```python
from build123d import *

# Parameters (mm, degrees)
BOSS_EXTRUDE1_DEPTH         = 561.975
F_1_4_20_TAPPED_HOLE1_D     = 5.1054
F_1_4_20_TAPPED_HOLE1_DEPTH = 16.51
F_1_4_20_TAPPED_HOLE1_TIP   = 1.533816902
F_1_4_20_TAPPED_HOLE2_D     = 5.1054
F_1_4_20_TAPPED_HOLE2_DEPTH = 16.51
F_1_4_20_TAPPED_HOLE2_TIP   = 1.533816902


with BuildPart() as part:
    # Sketch1 → Boss-Extrude1 (new body)
    with BuildSketch(Plane.XY):
        Polygon((7.332348419, 0), (3.666174209, 6.35), (-3.666174209, 6.35), (-7.332348419, 0), (-3.666174209, -6.35), (3.666174209, -6.35), align=None)
    extrude(amount=BOSS_EXTRUDE1_DEPTH)

    # 1/4-20 Tapped Hole1
    with Locations(Plane.XY.offset(561.975)):
        with Locations((0, 0)):
            Hole(F_1_4_20_TAPPED_HOLE1_D / 2, depth=F_1_4_20_TAPPED_HOLE1_DEPTH)
            with Locations((0, 0, -(F_1_4_20_TAPPED_HOLE1_DEPTH + F_1_4_20_TAPPED_HOLE1_TIP / 2))):  # 118° drill point
                Cone(0, F_1_4_20_TAPPED_HOLE1_D / 2, F_1_4_20_TAPPED_HOLE1_TIP, mode=Mode.SUBTRACT)

    # 1/4-20 Tapped Hole2
    with Locations(Plane(origin=(0, 0, 0), x_dir=(-1, 0, 0), z_dir=(0, 0, -1))):
        with Locations((0, 0)):
            Hole(F_1_4_20_TAPPED_HOLE2_D / 2, depth=F_1_4_20_TAPPED_HOLE2_DEPTH)
            with Locations((0, 0, -(F_1_4_20_TAPPED_HOLE2_DEPTH + F_1_4_20_TAPPED_HOLE2_TIP / 2))):  # 118° drill point
                Cone(0, F_1_4_20_TAPPED_HOLE2_D / 2, F_1_4_20_TAPPED_HOLE2_TIP, mode=Mode.SUBTRACT)


solid = part.part
```
Source: CAD feature listing. Evaluate the final solid. Frame: model axes, mm. Round coordinates to 2 decimals unless told otherwise and drop trailing zeros. Loops run counter-clockwise (first coordinate to the right, second up) from the corner with the lowest first, then second, coordinate; pieces in that order, holes last. Notation, with made-up numbers: M 15,-15 L 45,-15 A15 ccw 45,0 Z; hole C 42,-40 d2. An arc over 180 degrees is marked long. Use a Markdown table: item, result. Add a question column.
1. Contact query for a flat-ended pin moving along its axis: pin 1 (3 mm diameter, centred on x = 0, y = 0, fed in from +Z). Output: stop coordinate, or through.
2. Cut plane A-A, the plane z = 207. Output: boundary loops of the cut face in (x, y).
3. Ray query, line 1 along X through (y, z) = (0, 553.25); line 2 along Y through (x, z) = (0, 4.75); line 3 along X through (y, z) = (-1.75, 458.5). Return the intervals inside material, ascending. Write a range as [from, to].
Solution:
| question | item | result |
|---|---|---|
| 1 | pin 1 | stops at z = 544.83 |
| 2 | outline | M -7.33,0 L -3.67,-6.35 L 3.67,-6.35 L 7.33,0 L 3.67,6.35 L -3.67,6.35 Z |
| 3 | line 1 | x = [-7.33, -2.55], [2.55, 7.33] |
| 3 | line 2 | y = [-6.35, -2.55], [2.55, 6.35] |
| 3 | line 3 | x = [-6.32, 6.32] |
